from build123d import *

# Parameters (mm, degrees)
F2_DEPTH      = 2
F2_DEPTH_BACK = 6.4
F3_W          = 32.5771644663
F3_H          = 4.4
F4_DEPTH      = 56.5738534806
F7_DEPTH      = 19.1421356237
F7_DEPTH_BACK = 19.1421356237
F9_DEPTH      = 2
F0_R          = 2.75
F10_DEPTH     = 0.8
F11_R         = 0.4
F12_R         = 1
F13_R         = 5


with BuildPart() as f2:
    # F1 (on Top) → F2 (new body, two sides)
    with BuildSketch(Plane.XY) as f2_sk:
        Polygon((-8.7928932188, -35.8639610307), (17.0710678119, -10), (-10, 17.0710678119), (-35.8639610307, -8.7928932188), align=None)
    extrude(amount=F2_DEPTH)
    extrude(f2_sk.sketch, amount=-F2_DEPTH_BACK)

    # F3 (on face) → F4 (cut, through all)
    with BuildSketch(Plane(origin=(13.5355339059, -13.5355339059, 0), x_dir=(0.7071067812, 0.7071067812, 0), z_dir=(0.7071067812, -0.7071067812, 0))):
        with Locations((-11.2885822331, -2.2)):
            Rectangle(F3_W, F3_H)
    extrude(amount=-F4_DEPTH, mode=Mode.SUBTRACT)

    # F6 (on face) → F7 (join, two sides)
    with BuildSketch(Plane(origin=(0, 0, 0), x_dir=(0.7071067812, 0.7071067812, 0), z_dir=(0.7071067812, -0.7071067812, 0))) as f7_sk:
        with BuildLine():
            Line((-23.5771644663, 2), (-20.5771644663, 2))
            ThreePointArc((-20.5771644663, 2), (-22.9887071982, 11), (-29.5771644663, 17.5884572681))
            Line((-29.5771644663, 17.5884572681), (-31.0771644663, 14.9903810568))
            ThreePointArc((-31.0771644663, 14.9903810568), (-25.5867834095, 9.5), (-23.5771644663, 2))
        make_face()
    extrude(amount=-F7_DEPTH)
    extrude(f7_sk.sketch, amount=F7_DEPTH_BACK)

    # F8 (on face) → F9 (cut, through all)
    with BuildSketch(Plane(origin=(0, 0, -6.4), x_dir=(1, 0, 0), z_dir=(0, 0, -1))):
        Polygon((17.0710678119, 10), (-2, 29.0710678119), (-2, 2), (-29.0710678119, 2), (-10, -17.0710678119), align=None)
    extrude(amount=-F9_DEPTH, mode=Mode.SUBTRACT)

    # F0 (on Top) → F10 (join)
    with BuildSketch(Plane.XY):
        with Locations((10, -10)):
            Circle(F0_R)
        with Locations((-10, 10)):
            Circle(F0_R)
    extrude(amount=-F10_DEPTH)

    # F11
    f11_edges = [f2.edges().sort_by_distance(p)[0] for p in [
        (7.25, -10, -0.8),
        (-12.75, 10, -0.8),
    ]]
    fillet(f11_edges, radius=F11_R)

    # F12
    f12_edges = [f2.edges().sort_by_distance(p)[0] for p in [
        (-21.974874, -21.974874, 14.990381),
        (-20.914214, -20.914214, 17.588457),
        (-22.328427, -22.328427, 2),
        (-22.328427, -22.328427, -6.4),
    ]]
    fillet(f12_edges, radius=F12_R)

    # F13
    f13_edges = [f2.edges().sort_by_distance(p)[0] for p in [
        (17.071068, -10, 1),
        (-10, 17.071068, 1),
    ]]
    fillet(f13_edges, radius=F13_R)


solid = f2.part
CAD build for the part. Positions are in the model's coordinates, mm. A direction names the side the tool comes from. Give positions to 0.01 mm unless a question says otherwise; leave off trailing zeros. Loops run counter-clockwise (first coordinate to the right, second up) from the corner with the lowest first, then second, coordinate; pieces in that order, holes last. Notation, with made-up numbers: M -31,59 L 19,59 A21 ccw 19,65 Z; hole C 45,-14 d10. An arc over 180 degrees is marked long. One line per question, with ' | ' between items. Start each with the question number.
1. Saw through at A-A on x = 10. Give the cut face in (y, z), plus the area to 3 significant figures.
2. Probe L1, parallel to Z at x = -17.5, y = -17; L2, parallel to Z at x = -12, y = 5; L3, parallel to X at y = -28.5, z = -3.75. List the from-to ranges inside material, lowest first. Write a range as from..to.
3. Flat gauge pins, fed straight in: pin 1 (1.5 mm diameter, centred on y = -1, z = 0.5, fed in from -X); pin 2 (1 mm diameter, centred on y = -24, z = 1.5, fed in from +X); pin 3 (15.5 mm diameter, centred on x = -10.5, y = -14.5, fed in from +Z). Where does each tip first touch, or does it go through?
4. Saw through at C-C on z = 6. Give the cut face in (x, y).
5. 3-axis set-ups, long thin cutter, end or side, ignore diameter. For faces 1 (the face through (-8, -8, 0)), 2 (the face through (-15, -2, -5)), 3 (the face through (-18, -19, 2)), 4 (the face through (10, -10, -0.8)): which of +Z, -Z, +X, -X, +Y, -Y reach the whole face in a straight line?
6. Two-plate mould, pull along X, no slides. Class faces 5 (the face through (12.62, -9.17, -0.2)), 6 (the face through (-22.518, -22.139, -2.155)), 7 (the face through (15, -10, 1)): pulls with the +X half, pulls with the -X half, needs draft (parallel to the pull), parting line crosses it, or undercut.
Result sheet:
1) outline: M -17.07,0 L -12.75,0 L -12.75,-0.4 A0.4 ccw -12.35,-0.8 L -7.65,-0.8 A0.4 ccw -7.25,-0.4 L -7.25,0 L -2.93,0 L -2.93,2 L -17.07,2 Z | area: 32.6 mm^2
2) L1: z = -6.4..-4.4, 0..2, 6.89..13.08 | L2: z = 0..2 | L3: x = -16.16..-10.5
3) pin 1: stops at x = -28.82 | pin 2: stops at x = 3.57 | pin 3: stops at z = 14.29
4) outline: M -30.59,-3.52 L -3.52,-30.59 L -1.33,-28.4 L -28.4,-1.33 Z
5) face 1: none | face 2: -Z, +X, -X, +Y | face 3: -X, -Y | face 4: -Z, +X, +Y, -Y
6) face 5: undercut | face 6: pulls with the -X half | face 7: pulls with the +X half
